```python
from build123d import *

# Parameters (mm, degrees)
ESQUISSE1_W             = 15.712671493
ESQUISSE1_H             = 32.57240809
ESQUISSE1_R             = 1.2
BOSS_EXTRU_1_DEPTH      = 4
BOSS_EXTRU_2_DEPTH      = 10
BOSS_EXTRU_2_DEPTH_BACK = 16
BOSS_EXTRU_4_DEPTH      = 4


with BuildPart() as part:
    # Esquisse1 → Boss.-Extru.1 (new body)
    with BuildSketch(Plane.XY):
        with Locations((7.856335747, 16.286204045)):
            Rectangle(ESQUISSE1_W, ESQUISSE1_H)
        with Locations((7.85, 28.978207996)):
            Circle(ESQUISSE1_R, mode=Mode.SUBTRACT)
        with Locations((7.814879524, 18.978269669)):
            Circle(ESQUISSE1_R, mode=Mode.SUBTRACT)
    extrude(amount=BOSS_EXTRU_1_DEPTH)

    # Esquisse2 → Boss.-Extru.2 (add, two sides: drawn at the far end of the back side and taken through both)
    with BuildSketch(Plane.XZ.offset(-BOSS_EXTRU_2_DEPTH_BACK)):
        Polygon((-5.143664254, 4), (20.856335746, 4), (20.856335746, -8), (16.056335746, -8), (16.056335746, -3.5), (18.56763753, -3.5), (18.56763753, -0.5), (15.713373902, -0.5), (15.712671493, 0), (0, 0), (-0.00070241, -0.5), (-2.854966038, -0.5), (-2.854966038, -3.5), (-0.343664254, -3.5), (-0.343664254, -8), (-5.143664254, -8), align=None)
    extrude(amount=BOSS_EXTRU_2_DEPTH + BOSS_EXTRU_2_DEPTH_BACK)

    # Esquisse4 → Boss.-Extru.4 (add)
    with BuildSketch(Plane.XY.offset(4)):
        Polygon((0, 16), (-5.143664254, 16), (-5.143664254, 39.452985167), (20.856335746, 39.452985167), (20.856335746, 16), (15.712671493, 16), (14.344424764, 16), (14.344424764, 31.44629888), (1.552132881, 31.44629888), (1.552132881, 16), align=None)
    extrude(amount=-BOSS_EXTRU_4_DEPTH)


solid = part.part
```
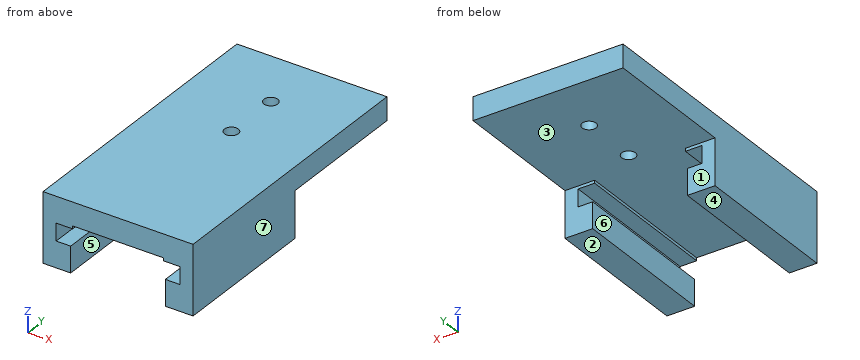
Design review of the part built by this model. Coordinates are the model's own, in mm. Face numbers are marked on the shaded views. A direction names the side the tool comes from. Give positions to 0.01 mm unless a question says otherwise; leave off trailing zeros. Loops run counter-clockwise (first coordinate to the right, second up) from the corner with the lowest first, then second, coordinate; pieces in that order, holes last. Notation, with made-up numbers: M 60,-3 L 105,-3 A26 cw 105,31 Z; hole C 4,11 d7. An arc over 180 degrees is marked long. Return JSON: item names as keys, results as strings. Group by question number.
Item 1: Tool access review of the marked faces 1, 2 and 3: name each direction out of +Z, -Z, +X, -X, +Y, -Y from which nothing blocks a thin tool from reaching the whole face with its end or side.
Item 2: We need section A-A (z = -5). Give the boundary of the cut face in (x, y), and give its area (3 significant figures).
Item 3: We need section C-C (y = 11.5). Give the boundary of the cut face in (x, z), and give its area (3 significant figures).
Item 4: We need section B-B (x = -1.5). Give the boundary of the cut face in (y, z), and give its area (3 significant figures).
Item 5: We need section D-D (x = 7.85). Give the boundary of the cut face in (y, z).
Item 6: Insertion check: pin 1 Ø4 at (x, z) = (18.5, -2.5) entering from +Y; pin 2 Ø4 at (x, y) = (7.85, 28.98) entering from +Z; pin 3 Ø2 at (x, y) = (7.81, 18.98) entering from +Z; pin 4 Ø13 at (x, y) = (12, 27) entering from -Z. Each pin has a flat end and moves straight along its axis. Give the tip position at first contact, or say it passes through.
Item 7: Mouldability with a two-part tool opening along X and no side actions: class the marked faces 4, 5, 6 and 7 as released by +X, released by -X, zero draft, split by the parting line, or undercut.
Item 8: For probe 1 along Y at (x, z) = (7.85, 2.9); probe 2 along X at (y, z) = (2, -7); probe 3 along Z at (x, y) = (17.75, 15), list the stretches that pass through material, from the lowest coordinate up.
Output:
{
 "1": {"face 1": "-Z, +X, -X, +Y", "face 2": "-Z, +X, -X, +Y, -Y", "face 3": "-Z, +Y"},
 "2": {"outline": "M -5.14,-10 L -0.34,-10 L -0.34,16 L -5.14,16 Z; M 16.06,-10 L 20.86,-10 L 20.86,16 L 16.06,16 Z", "area": "250 mm^2"},
 "3": {"outline": "M -5.14,-8 L -0.34,-8 L -0.34,-3.5 L -2.85,-3.5 L -2.85,-0.5 L 0,-0.5 L 0,0 L 15.71,0 L 15.71,-0.5 L 18.57,-0.5 L 18.57,-3.5 L 16.06,-3.5 L 16.06,-8 L 20.86,-8 L 20.86,4 L -5.14,4 Z", "area": "166 mm^2"},
 "4": {"outline": "M -10,-8 L 16,-8 L 16,-3.5 L -10,-3.5 Z; M -10,-0.5 L 16,-0.5 L 16,0 L 39.45,0 L 39.45,4 L -10,4 Z", "area": "328 mm^2"},
 "5": {"outline": "M -10,0 L 17.78,0 L 17.78,4 L -10,4 Z; M 20.18,0 L 27.78,0 L 27.78,4 L 20.18,4 Z; M 30.18,0 L 39.45,0 L 39.45,4 L 30.18,4 Z"},
 "6": {"pin 1": "stops at y = 16", "pin 2": "stops at z = 4", "pin 3": "passes through", "pin 4": "stops at z = 0"},
 "7": {"face 4": "zero draft", "face 5": "undercut", "face 6": "undercut", "face 7": "released by +X"},
 "8": {"probe 1": "y = -10 to 17.78, 20.18 to 27.78, 30.18 to 39.45", "probe 2": "x = -5.14 to -0.34, 16.06 to 20.86", "probe 3": "z = -8 to -3.5, -0.5 to 4"}
}
